Build history of the part. All positions in model axes, mm. A direction names the side the tool comes from. Give positions to 0.01 mm unless a question says otherwise; leave off trailing zeros. Order: outer loops, then holes, each group sorted by start corner. A loop starts at its lowest first (then second) coordinate and runs counter-clockwise, first axis right, second up. Notation, with made-up numbers: (69, 72) - (121, 72) arc R16 cw to (121, 97) - close; hole circle Ø6 at (-35.5, 64). An arc over 180 degrees is marked (long way). One line per item, written item: value.
```python
from build123d import *

# Parameters (mm, degrees)
SKETCH_1_R               = 5.9
SKETCH_1_R_2             = 3.4
EXTRUDE_1_DEPTH          = 8
PATTERN_CIRCULAR_1_COUNT = 2


with BuildPart() as part:
    # 스케치1 → 보스-돌출1 (new body)
    with BuildSketch(Plane.XY):
        Circle(SKETCH_1_R)
        Circle(SKETCH_1_R_2, mode=Mode.SUBTRACT)
    extrude(amount=EXTRUDE_1_DEPTH)

    # 스케치6 → M2 남비 머리 나사용 카운터보어3 (revolve, cut)
    with BuildSketch(Plane(origin=(0, 5.9, 4), x_dir=(0, 0, 1), z_dir=(1, 0, 0))):
        Polygon((0, 0), (0, 5.781118805), (1.3, 5), (1.3, 1.6), (2.5, 1.6), (2.5, 0), align=None)
    hole_wizard_m2_3 = revolve(axis=Axis((0, 12.25, 4), (0, -1, 0)), mode=Mode.SUBTRACT)

    # 원형 패턴1: M2 남비 머리 나사용 카운터보어3 ×2 about axis
    pattern_circular_1_axis = Axis((0, 0, 8), (0, 0, 1))
    for i in range(1, PATTERN_CIRCULAR_1_COUNT):
        add(hole_wizard_m2_3.rotate(pattern_circular_1_axis, i * 360 / PATTERN_CIRCULAR_1_COUNT), mode=Mode.SUBTRACT)


solid = part.part
```
(1) Pull direction Z, two halves, no side cores. Call faces 1 (the face through (0.79, 3.73, 2.97)), 2 (the face through (3, -3, 0)), 3 (the face through (3, -3, 8)): +Z half, -Z half, draft (parallel to the pull), parting line (faces both ways), or undercut.
Completed:
face 1: undercut
face 2: -Z half
face 3: +Z half
(2) Slice it at D-D, the plane x = -2. Give the cut face in (y, z).
Completed:
outline: (-5.55, 0) - (-2.75, 0) - (-2.75, 8) - (-5.55, 8) - (-5.55, 5.5) - (-4.3, 5.5) - (-4.3, 2.5) - (-5.55, 2.5) - close; (2.75, 0) - (5.55, 0) - (5.55, 2.5) - (4.3, 2.5) - (4.3, 5.5) - (5.55, 5.5) - (5.55, 8) - (2.75, 8) - close
(3) Drill centre lines: line 1 (Z direction, x = 0, y = 3.85); line 2 (Z direction, x = 0, y = 5.35); line 3 (Y direction, x = -2, z = 5.75). Where is each one in solid material? Low to high.
Completed:
line 1: 0 to 2.7, 5.3 to 8
line 2: 0 to 1.5, 6.5 to 8
line 3: -5.55 to -2.75, 2.75 to 5.55
(4) Pin check, flat tips, straight feed: P1, Ø1, axis at x = -4.5, z = 3, coming from the -Y side; P2, Ø1.5, axis at x = 2.5, y = 1.5, coming from the +Z side; P3, Ø1.5, axis at y = -1.5, z = 1, coming from the -X side; P4, Ø1.5, axis at x = 2.5, z = 1, coming from the -Y side. Stop position of each tip, or through.
Completed:
P1: y = -4.34
P2: z = 8
P3: x = -5.85
P4: y = -5.63
(5) Slice it at A-A, the plane x = 0. Give the cut face in (y, z).
Completed:
outline: (-5.9, 0) - (-3.4, 0) - (-3.4, 2.7) - (-4.3, 2.7) - (-4.3, 1.5) - (-5.9, 1.5) - close; (-5.9, 6.5) - (-4.3, 6.5) - (-4.3, 5.3) - (-3.4, 5.3) - (-3.4, 8) - (-5.9, 8) - close; (3.4, 0) - (5.9, 0) - (5.9, 1.5) - (4.3, 1.5) - (4.3, 2.7) - (3.4, 2.7) - close; (3.4, 5.3) - (4.3, 5.3) - (4.3, 6.5) - (5.9, 6.5) - (5.9, 8) - (3.4, 8) - close
(6) Slice it at B-B, the plane y = 0. Give the cut face in (x, z), and give its area (3 significant figures).
Completed:
outline: (-5.9, 0) - (-3.4, 0) - (-3.4, 8) - (-5.9, 8) - close; (3.4, 0) - (5.9, 0) - (5.9, 8) - (3.4, 8) - close
area: 40.0 mm²
(7) 3-axis set-ups, long thin cutter, end or side, ignore diameter. For faces 4 (the face through (-0.79, -3.73, 2.97)), 5 (the face through (-1.69, 4.93, 2.16)), 6 (the face through (1.69, -4.93, 2.16)): which of +Z, -Z, +X, -X, +Y, -Y reach the whole face in a straight line?
Completed:
face 4: +Y, -Y
face 5: +Y
face 6: -Y
(8) Slice it at C-C, the plane z = 3.75. Give the cut face in (x, y), and give its area (3 significant figures).
Completed:
outline: (-2.49, -5.35) - (-2.49, -4.3) - (-1.28, -4.3) - (-1.28, -3.15) arc R3.4 cw to (-1.28, 3.15) - (-1.28, 4.3) - (-2.49, 4.3) - (-2.49, 5.35) arc R5.9 ccw to start; (1.28, -4.3) - (2.49, -4.3) - (2.49, -5.35) arc R5.9 ccw to (2.49, 5.35) - (2.49, 4.3) - (1.28, 4.3) - (1.28, 3.15) arc R3.4 cw to (1.28, -3.15) - close
area: 53.9 mm²
